Geometry: see drawing. Coordinates: mm, zero at the bounding-box minimum. Coordinates: 2 decimals unless noted, no trailing zeros. Loops run counter-clockwise (first coordinate to the right, second up) from the corner with the lowest first, then second, coordinate; pieces in that order, holes last.
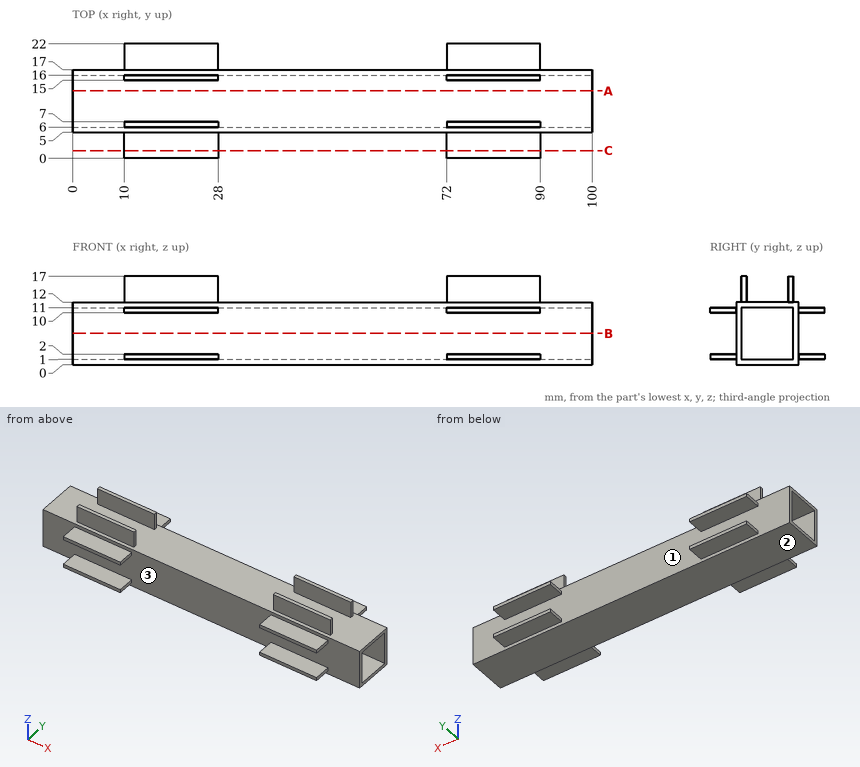
Item 1: Section query A-A (y = 13). Output: boundary loops of the cut face in (x, z).
Result:
outline: (0, 0) - (100, 0) - (100, 1) - (0, 1) - close; (0, 11) - (100, 11) - (100, 12) - (0, 12) - close
Item 2: Contact query for flat-ended pins moving along their axis: P1, Ø1, axis at x = 54.5, z = 10, coming from the +Y side; P2, Ø1.5, axis at x = 63.5, z = 13.5, coming from the -Y side; P3, Ø1.5, axis at x = 15.5, y = 20.5, coming from the +Z side; P4, Ø4, axis at x = 20, y = 2.5, coming from the -Z side. Output: stop coordinate, or through.
Result:
P1: stops at y = 17
P2: passes through
P3: stops at z = 11
P4: stops at z = 1
Item 3: Section query C-C (y = 1.5). Output: boundary loops of the cut face in (x, z), then the cut area to 3 significant figures.
Result:
outline: (10, 1) - (28, 1) - (28, 2) - (10, 2) - close; (10, 10) - (28, 10) - (28, 11) - (10, 11) - close; (72, 1) - (90, 1) - (90, 2) - (72, 2) - close; (72, 10) - (90, 10) - (90, 11) - (72, 11) - close
area: 72.0 mm2
Item 4: Mould query, pull axis Z, two halves, no side actions, for the marked faces 1, 2 and 3. Classes: +Z half, -Z half, draft (parallel to the pull), parting line (faces both ways), or undercut.
Result:
face 1: undercut
face 2: -Z half
face 3: undercut
Item 5: Line query: L1, parallel to Y at x = 81, z = 15.25; L2, parallel to Z at x = 17.5, y = 2.5; L3, parallel to Z at x = 83.5, y = 14. Output: solid intervals per line, ascending.
Result:
L1: y = 6 to 7, 15 to 16
L2: z = 1 to 2, 10 to 11
L3: z = 0 to 1, 11 to 12
Item 6: Section query B-B (z = 6). Output: boundary loops of the cut face in (x, y), then the cut area to 3 significant figures.
Result:
outline: (0, 5) - (100, 5) - (100, 6) - (0, 6) - close; (0, 16) - (100, 16) - (100, 17) - (0, 17) - close
area: 200 mm2
